Geometry: final body of the model. Coordinates: model frame, mm. Round coordinates to 2 decimals unless told otherwise and drop trailing zeros. Loops run counter-clockwise (first coordinate to the right, second up) from the corner with the lowest first, then second, coordinate; pieces in that order, holes last. Notation, with made-up numbers: (36.5, 44.5) - (47.5, 44.5) arc R22 ccw to (47.5, 74.5) - close; hole circle Ø11 at (-12, 67). An arc over 180 degrees is marked (long way). Write item = value, one per line. Start each with the question number.
Item 1: Section B-B (y = -587). Return loops of the section in (x, z).
Item 2: Section C-C (x = 138). Return loops of the section in (y, z).
Item 3: First-contact query: pin 1 (8 mm diameter, centred on x = -144, z = -4, fed in from -Y); pin 2 (1.9 mm diameter, centred on x = -533.4, y = -739.775, fed in from +Z); pin 3 (5 mm diameter, centred on x = -13.5, z = -9, fed in from -Y); pin 4 (2 mm diameter, centred on x = 514.5, z = -11, fed in from -Y). Flat tips, straight axial feed; report the tip coordinate or a pass-through.
Item 4: Line query: line 1 (X direction, y = 520.7, z = -9.75); line 2 (X direction, y = 342.9, z = -14.5); line 3 (Y direction, x = -533.4, z = -9.5). Output: solid intervals per line, ascending. Write a range as from..to.
Item 5: Section A-A (z = -15.5). Count the separate pieces of the cut face and the enclosed holes in it, plus the area to 3 significant figures.
from build123d import *

# Parameters (mm, degrees)
F0_R     = 1.5875
F1_DEPTH = 19.05
F2_R     = 6.35
F3_R     = 7.9375
F4_DEPTH = 6.35


with BuildPart() as f1:
    # F0 (on Top) → F1 (new body)
    with BuildSketch(Plane.XY):
        with BuildLine():
            Line((-571.5, 571.5), (-571.5, -749.3))
            Line((-571.5, -749.3), (-215.9, -749.3))
            ThreePointArc((-215.9, -749.3), (-206.919744, -745.580256), (-203.2, -736.6))
            Line((-203.2, -736.6), (-203.2, 0))
            ThreePointArc((-203.2, 0), (-143.684098, 143.684098), (0, 203.2))
            Line((0, 203.2), (635, 203.2))
            ThreePointArc((635, 203.2), (643.980256, 206.919744), (647.7, 215.9))
            Line((647.7, 215.9), (647.7, 571.5))
            Line((647.7, 571.5), (-571.5, 571.5))
        make_face()
        with Locations((-533.4, -739.775)):
            Circle(F0_R, mode=Mode.SUBTRACT)
        with Locations((-561.975, -698.5)):
            Circle(F0_R, mode=Mode.SUBTRACT)
        with Locations((-381, -739.775)):
            Circle(F0_R, mode=Mode.SUBTRACT)
        with Locations((-561.975, -419.1)):
            Circle(F0_R, mode=Mode.SUBTRACT)
        with Locations((-254, -739.775)):
            Circle(F0_R, mode=Mode.SUBTRACT)
        with Locations((-561.9877, -88.9)):
            Circle(F0_R, mode=Mode.SUBTRACT)
        with Locations((-561.975, 241.3)):
            Circle(F0_R, mode=Mode.SUBTRACT)
        with Locations((-342.9, 139.7)):
            Circle(F0_R, mode=Mode.SUBTRACT)
        with Locations((-342.9, 342.9)):
            Circle(F0_R, mode=Mode.SUBTRACT)
        with Locations((-561.975, 520.7)):
            Circle(F0_R, mode=Mode.SUBTRACT)
        with Locations((-520.7, 520.7)):
            Circle(F0_R, mode=Mode.SUBTRACT)
        with Locations((-520.7, 561.975)):
            Circle(F0_R, mode=Mode.SUBTRACT)
        with Locations((-266.7, 561.975)):
            Circle(F0_R, mode=Mode.SUBTRACT)
        with Locations((38.1, 561.975)):
            Circle(F0_R, mode=Mode.SUBTRACT)
        with Locations((638.175, 254)):
            Circle(F0_R, mode=Mode.SUBTRACT)
        with Locations((638.175, 387.35)):
            Circle(F0_R, mode=Mode.SUBTRACT)
        with Locations((342.9, 561.975)):
            Circle(F0_R, mode=Mode.SUBTRACT)
        with Locations((638.175, 520.7)):
            Circle(F0_R, mode=Mode.SUBTRACT)
        with Locations((596.9, 561.975)):
            Circle(F0_R, mode=Mode.SUBTRACT)
    extrude(amount=-F1_DEPTH)

    # F2
    f2_edges = [f1.edges().sort_by_distance(p)[0] for p in [
        (-393.7, -749.3, 0),
    ]]
    fillet(f2_edges, radius=F2_R)

    # F3 (on face) → F4 (cut)
    with BuildSketch(Plane.XY):
        with Locations((-342.9, 342.9)):
            Circle(F3_R)
    extrude(amount=-F4_DEPTH, mode=Mode.SUBTRACT)


solid = f1.part
Taken from the geometry:
q1.outline = (-571.5, -19.05) - (-203.2, -19.05) - (-203.2, -6.35) arc R6.35 ccw to (-209.55, 0) - (-571.5, 0) - close
q2.outline = (203.2, -19.05) - (571.5, -19.05) - (571.5, 0) - (209.55, 0) arc R6.35 ccw to (203.2, -6.35) - close
q3.pin_1 = 139.58
q3.pin_2 = through
q3.pin_3 = 202.57
q3.pin_4 = 203.2
q4.line_1 = -571.5..-563.56, -560.39..-522.29, -519.11..636.59, 639.76..647.7
q4.line_2 = -571.5..-344.49, -341.31..647.7
q4.line_3 = -749.3..-741.36, -738.19..571.5
q5.separate_pieces = 1
q5.enclosed_holes = 19
q5.area = 808,000 mm^2
